Check sheet for the modelled part. Datum: model origin and axes. Units: mm. Face numbers are marked on the shaded views. Round coordinates to 2 decimals unless told otherwise and drop trailing zeros. Loops run counter-clockwise (first coordinate to the right, second up) from the corner with the lowest first, then second, coordinate; pieces in that order, holes last. Notation, with made-up numbers: (-35, -2) - (21, -2) arc R8 cw to (21, 11) - close; hole circle Ø8 at (-28, 58.5). An arc over 180 degrees is marked (long way). Answer in a Markdown table with one row per item. Add a question column.
(1) Cross-section at A-A on x = 0. Enter the section's corners in (y, z) (1 decimal), then the cut area to 3 significant figures.
(2) Mould release check, pull along Y, two halves, no side actions. Record for the marked faces 1, 2 and 3: +Y half, -Y half, draft (parallel to the pull), parting line (faces both ways), or undercut.
(3) Thickness scan on line 1 along X through (y, z) = (8, 0.6); line 2 along Y through (x, z) = (5, 2.6); line 3 along Y through (x, z) = (-12, 1.1). Record the ranges inside material, lowest first.
(4) Cross-section at C-C on x = -12. Enter the section's corners in (y, z) (1 decimal), then the cut area to 3 significant figures.
(5) Cross-section at D-D on z = 1. Count the separate pieces of the cut face and the enclosed holes in it, then the cut area to 3 significant figures.
(6) Gauge pin test, flat ends, axial feed: pin 1 (6.5 mm diameter, centred on x = -12.35, y = -12.35, fed in from +Z); pin 2 (1.5 mm diameter, centred on x = 15, z = 2, fed in from +Y); pin 3 (1 mm diameter, centred on x = -4, z = 1.5, fed in from -Y). Record the tip position at first contact, or that the pin passes through.
from build123d import *

# Parameters (mm, degrees)
F0_R     = 23.01875
F0_R_2   = 3.96875
F0_R_3   = 2.15265
F0_R_4   = 11.1125
F1_DEPTH = 3.175
F3_DEPTH = 3.175


with BuildPart() as f1:
    # F0 (on Top) → F1 (new body)
    with BuildSketch(Plane.XY):
        Circle(F0_R)
        with Locations((-12.347852, -12.347852)):
            Circle(F0_R_2, mode=Mode.SUBTRACT)
        with Locations((12.347852, -12.347852)):
            Circle(F0_R_3, mode=Mode.SUBTRACT)
        with Locations((-12.347852, 12.347852)):
            Circle(F0_R_3, mode=Mode.SUBTRACT)
        Circle(F0_R_4, mode=Mode.SUBTRACT)
        with Locations((12.347852, 12.347852)):
            Circle(F0_R_2, mode=Mode.SUBTRACT)
    extrude(amount=F1_DEPTH)

    # F2 (on face) → F3 (cut, through all)
    with BuildSketch(Plane.XY.offset(3.175)):
        with BuildLine():
            ThreePointArc((-9.771912, 17.270905), (-7.652597, 15.318794), (-6.795954, 12.567723))
            ThreePointArc((-6.795954, 12.567723), (0, 14.2875), (6.795954, 12.567723))
            ThreePointArc((6.795954, 12.567723), (7.652597, 15.318794), (9.771912, 17.270905))
            ThreePointArc((9.771912, 17.270905), (0, 19.84375), (-9.771912, 17.270905))
        make_face()
        with BuildLine():
            ThreePointArc((-12.567723, 6.795954), (-15.318794, 7.652597), (-17.270905, 9.771912))
            ThreePointArc((-17.270905, 9.771912), (-19.84375, 0), (-17.270905, -9.771912))
            ThreePointArc((-17.270905, -9.771912), (-15.318794, -7.652597), (-12.567723, -6.795954))
            ThreePointArc((-12.567723, -6.795954), (-14.2875, 0), (-12.567723, 6.795954))
        make_face()
        with BuildLine():
            ThreePointArc((17.270905, 9.771912), (15.318794, 7.652597), (12.567723, 6.795954))
            ThreePointArc((12.567723, 6.795954), (14.2875, 0), (12.567723, -6.795954))
            ThreePointArc((12.567723, -6.795954), (15.318794, -7.652597), (17.270905, -9.771912))
            ThreePointArc((17.270905, -9.771912), (19.84375, 0), (17.270905, 9.771912))
        make_face()
        with BuildLine():
            ThreePointArc((-6.795954, -12.567723), (-7.652597, -15.318794), (-9.771912, -17.270905))
            ThreePointArc((-9.771912, -17.270905), (0, -19.84375), (9.771912, -17.270905))
            ThreePointArc((9.771912, -17.270905), (7.652597, -15.318794), (6.795954, -12.567723))
            ThreePointArc((6.795954, -12.567723), (0, -14.2875), (-6.795954, -12.567723))
        make_face()
    extrude(amount=-F3_DEPTH, mode=Mode.SUBTRACT)


solid = f1.part
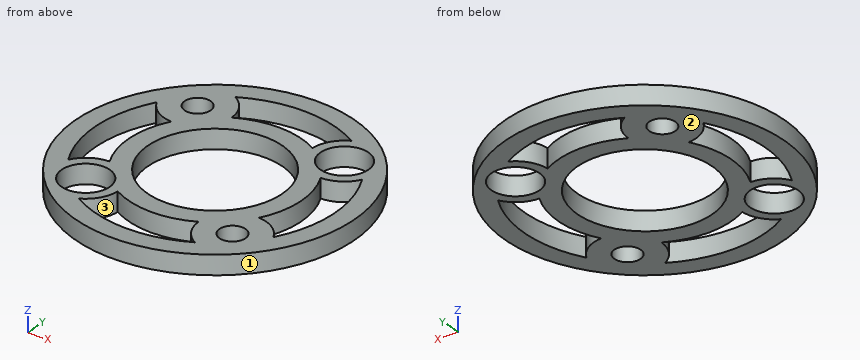
Answers:
| question | item | result |
|---|---|---|
| 1 | outline | (-23, 0) - (-19.8, 0) - (-19.8, 3.2) - (-23, 3.2) - close; (-14.3, 0) - (-11.1, 0) - (-11.1, 3.2) - (-14.3, 3.2) - close; (11.1, 0) - (14.3, 0) - (14.3, 3.2) - (11.1, 3.2) - close; (19.8, 0) - (23, 0) - (23, 3.2) - (19.8, 3.2) - close |
| 1 | area | 40.3 mm^2 |
| 2 | face 1 | parting line |
| 2 | face 2 | draft |
| 2 | face 3 | undercut |
| 3 | line 1 | x = -21.58 to -18.16, -15.81 to -7.71, 7.71 to 15.81, 18.16 to 21.58 |
| 3 | line 2 | y = -22.47 to -19.2, -13.38 to -9.92, 9.92 to 13.38, 19.2 to 22.47 |
| 3 | line 3 | y = -19.64 to -16.3, -8.39 to 10.22, 14.47 to 19.64 |
| 4 | outline | (-19.6, 0) - (-16.3, 0) - (-16.3, 3.2) - (-19.6, 3.2) - close; (-8.4, 0) - (10.2, 0) - (10.2, 3.2) - (-8.4, 3.2) - close; (14.5, 0) - (19.6, 0) - (19.6, 3.2) - (14.5, 3.2) - close |
| 4 | area | 86.1 mm^2 |
| 5 | separate pieces | 1 |
| 5 | enclosed holes | 9 |
| 5 | area | 787 mm^2 |
| 6 | pin 1 | passes through |
| 6 | pin 2 | stops at y = 18.08 |
| 6 | pin 3 | stops at y = -22.75 |
